Check sheet for the modelled part. Datum: model origin and axes. Units: mm. Face numbers are marked on the shaded views. Round coordinates to 2 decimals unless told otherwise and drop trailing zeros. Order: outer loops, then holes, each group sorted by start corner. A loop starts at its lowest first (then second) coordinate and runs counter-clockwise, first axis right, second up. Notation, with made-up numbers: (78, -32.75) -> (132, -32.75) arc R21 ccw to (132, -2.75) -> close; hole circle Ø1 at (-10.5, -30.75). An arc over 180 degrees is marked (long way). Answer in a Markdown table with one row per item.
from build123d import *

# Parameters (mm, degrees)
EXTRUDE_THIN1_DEPTH = 9.525


with BuildPart() as part:
    # Sketch1 → Extrude-Thin1 (new, symmetric)
    with BuildSketch(Plane(origin=(0, 0, 0), x_dir=(0, 0, -1), z_dir=(1, 0, 0))):
        with BuildLine():
            Line((-0.1778, 31.39), (-0.1778, 2.175027104))
            Line((-0.1778, 2.175027104), (-1.176413552, 1.176413552))
            ThreePointArc((-1.176413552, 1.176413552), (0, -1.6637), (1.176413552, 1.176413552))
            Line((1.176413552, 1.176413552), (0.1778, 2.175027104))
            Line((0.1778, 2.175027104), (0.1778, 19.05))
            Line((0.1778, 19.05), (0.0254, 19.05))
            Line((0.0254, 19.05), (0.0254, 2.111900957))
            Line((0.0254, 2.111900957), (1.068650478, 1.068650478))
            ThreePointArc((1.068650478, 1.068650478), (0, -1.5113), (-1.068650478, 1.068650478))
            Line((-1.068650478, 1.068650478), (-0.0254, 2.111900957))
            Line((-0.0254, 2.111900957), (-0.0254, 31.39))
            Line((-0.0254, 31.39), (-0.1778, 31.39))
        make_face()
    extrude(amount=EXTRUDE_THIN1_DEPTH, both=True)


solid = part.part
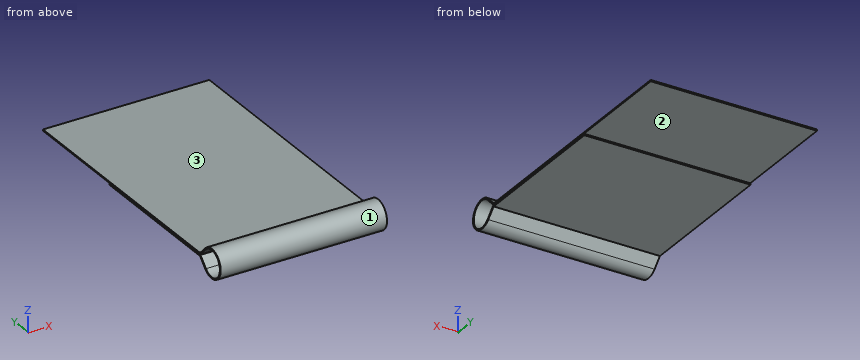
Item 1: Cross-section at A-A (y = 0). Record the boundary of the cut face in (x, z) (3 decimals), and give its area (3 significant figures).
Result sheet:
| item | result |
|---|---|
| outline | (-9.525, -1.664) -> (9.525, -1.664) -> (9.525, -1.511) -> (-9.525, -1.511) -> close; (-9.525, 1.511) -> (9.525, 1.511) -> (9.525, 1.664) -> (-9.525, 1.664) -> close |
| area | 5.81 mm^2 |
Item 2: Scan lines: line 1 (Z direction, x = 2, y = 0); line 2 (Y direction, x = -0.5, z = -1.35); line 3 (Y direction, x = -5, z = 1.25). Record each from-to range of solid material in increasing order. Write a range as [from, to].
Result sheet:
| item | result |
|---|---|
| line 1 | z = [-1.66, -1.51], [1.51, 1.66] |
| line 2 | y = [-0.97, -0.68], [0.68, 0.97] |
| line 3 | y = [-1.1, -0.85], [0.85, 1.1] |
Item 3: Cross-section at C-C (y = 29.5). Record the boundary of the cut face in (x, z) (3 decimals), and give its area (3 significant figures).
Result sheet:
| item | result |
|---|---|
| outline | (-9.525, 0.025) -> (9.525, 0.025) -> (9.525, 0.178) -> (-9.525, 0.178) -> close |
| area | 2.90 mm^2 |
Item 4: Depth check by flat-ended pin: P1, Ø1.5, axis at x = 2.5, z = -1, coming from the -Y side; P2, Ø5, axis at x = 2.5, y = 9.5, coming from the -Z side; P3, Ø8.5, axis at x = 0, y = 12.5, coming from the +Z side. Enter the tip coordinate at first touch or a pass-through.
Result sheet:
| item | result |
|---|---|
| P1 | stops at y = -1.64 |
| P2 | stops at z = -0.18 |
| P3 | stops at z = 0.18 |
Item 5: Cross-section at B-B (x = 1). Record the boundary of the cut face in (y, z).
Result sheet:
| item | result |
|---|---|
| outline | (1.07, -1.07) arc R1.51 cw (long way) to (1.07, 1.07) -> (2.11, 0.03) -> (31.39, 0.03) -> (31.39, 0.18) -> (2.18, 0.18) -> (1.18, 1.18) arc R1.66 ccw (long way) to (1.18, -1.18) -> (2.18, -0.18) -> (19.05, -0.18) -> (19.05, -0.03) -> (2.11, -0.03) -> close |
Item 6: Mould release check, pull along Z, two halves, no side actions. Record for the marked faces 1, 2 and 3: pulls with the +Z half, pulls with the -Z half, needs draft (parallel to the pull), parting line crosses it, or undercut.
Result sheet:
| item | result |
|---|---|
| face 1 | parting line crosses it |
| face 2 | undercut |
| face 3 | pulls with the +Z half |
